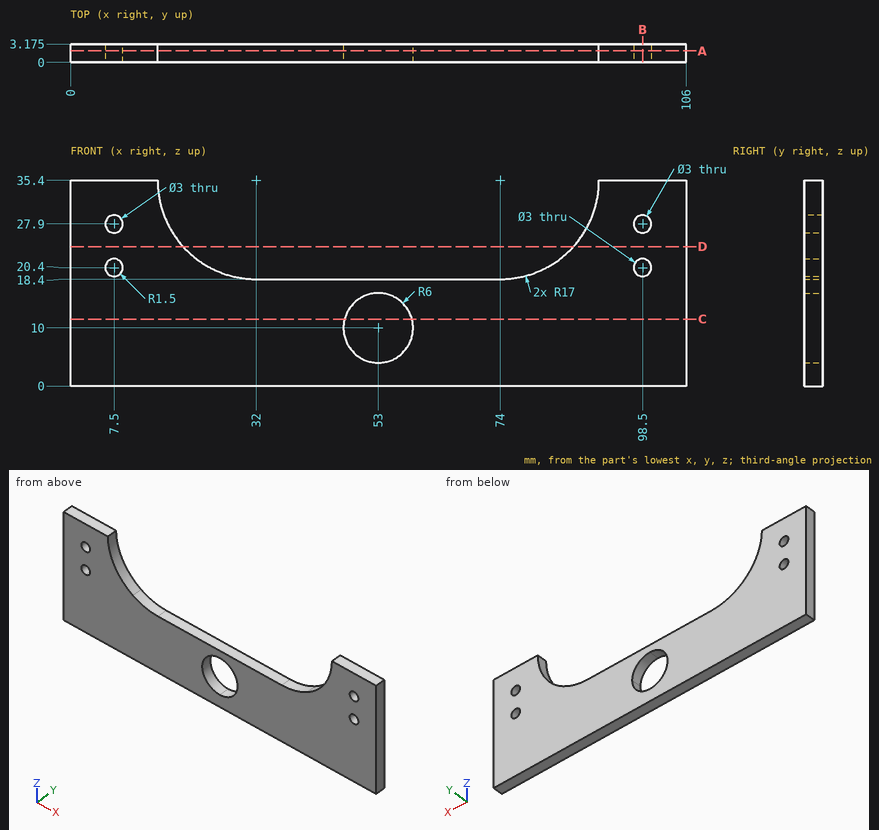
Verification items for this drawing (mm, ordinates from the low corner). Coordinates: 2 decimals unless noted, no trailing zeros. Loops run counter-clockwise (first coordinate to the right, second up) from the corner with the lowest first, then second, coordinate; pieces in that order, holes last. Notation, with made-up numbers: (51.25, 52) -> (60.25, 52) arc R23 ccw to (60.25, 69) -> close; hole circle Ø10 at (6.25, 12.25). An arc over 180 degrees is marked (long way). Answer in a Markdown table with one row per item. Add a question column.
1. Material ranges on probe 1 along Z at (x, y) = (98.5, 0.95); probe 2 along X at (y, z) = (2.55, 29); probe 3 along X at (y, z) = (1.2, 28), recorded low to high. Write a range as [from, to].
2. Section check A-A, the plane y = 2. Enter the section's corners in (x, z), then the cut area to 3 significant figures.
3. Section check B-B, the plane x = 98.5. Enter the section's corners in (y, z) (3 decimals), then the cut area to 3 significant figures.
4. Section check C-C, the plane z = 11.5. Enter the section's corners in (x, y) (3 decimals), then the cut area to 3 significant figures.
5. Section check D-D, the plane z = 24. Enter the section's corners in (x, y) (3 decimals), then the cut area to 3 significant figures.
Derived:
| question | item | result |
|---|---|---|
| 1 | probe 1 | z = [0, 18.9], [21.9, 26.4], [29.4, 35.4] |
| 1 | probe 2 | x = [0, 6.48], [8.52, 16.25], [89.75, 97.48], [99.52, 106] |
| 1 | probe 3 | x = [0, 6], [9, 16.7], [89.3, 97], [100, 106] |
| 2 | outline | (0, 0) -> (106, 0) -> (106, 35.4) -> (91, 35.4) arc R17 cw to (74, 18.4) -> (32, 18.4) arc R17 cw to (15, 35.4) -> (0, 35.4) -> close; hole circle Ø3 at (7.5, 20.4); hole circle Ø3 at (7.5, 27.9); hole circle Ø12 at (53, 10); hole circle Ø3 at (98.5, 20.4); hole circle Ø3 at (98.5, 27.9) |
| 2 | area | 2,440 mm² |
| 3 | outline | (0, 0) -> (3.175, 0) -> (3.175, 18.9) -> (0, 18.9) -> close; (0, 21.9) -> (3.175, 21.9) -> (3.175, 26.4) -> (0, 26.4) -> close; (0, 29.4) -> (3.175, 29.4) -> (3.175, 35.4) -> (0, 35.4) -> close |
| 3 | area | 93.3 mm² |
| 4 | outline | (0, 0) -> (47.191, 0) -> (47.191, 3.175) -> (0, 3.175) -> close; (58.809, 0) -> (106, 0) -> (106, 3.175) -> (58.809, 3.175) -> close |
| 4 | area | 300 mm² |
| 5 | outline | (0, 0) -> (19.389, 0) -> (19.389, 3.175) -> (0, 3.175) -> close; (86.611, 0) -> (106, 0) -> (106, 3.175) -> (86.611, 3.175) -> close |
| 5 | area | 123 mm² |
